Verification items for this drawing (mm, ordinates from the low corner). A direction names the side the tool comes from. Coordinates: 2 decimals unless noted, no trailing zeros. Write each loop counter-clockwise with the first axis right and the second up, starting at its lowest first coordinate (ties: lowest second). Pieces come first, ordered by that corner, then holes.
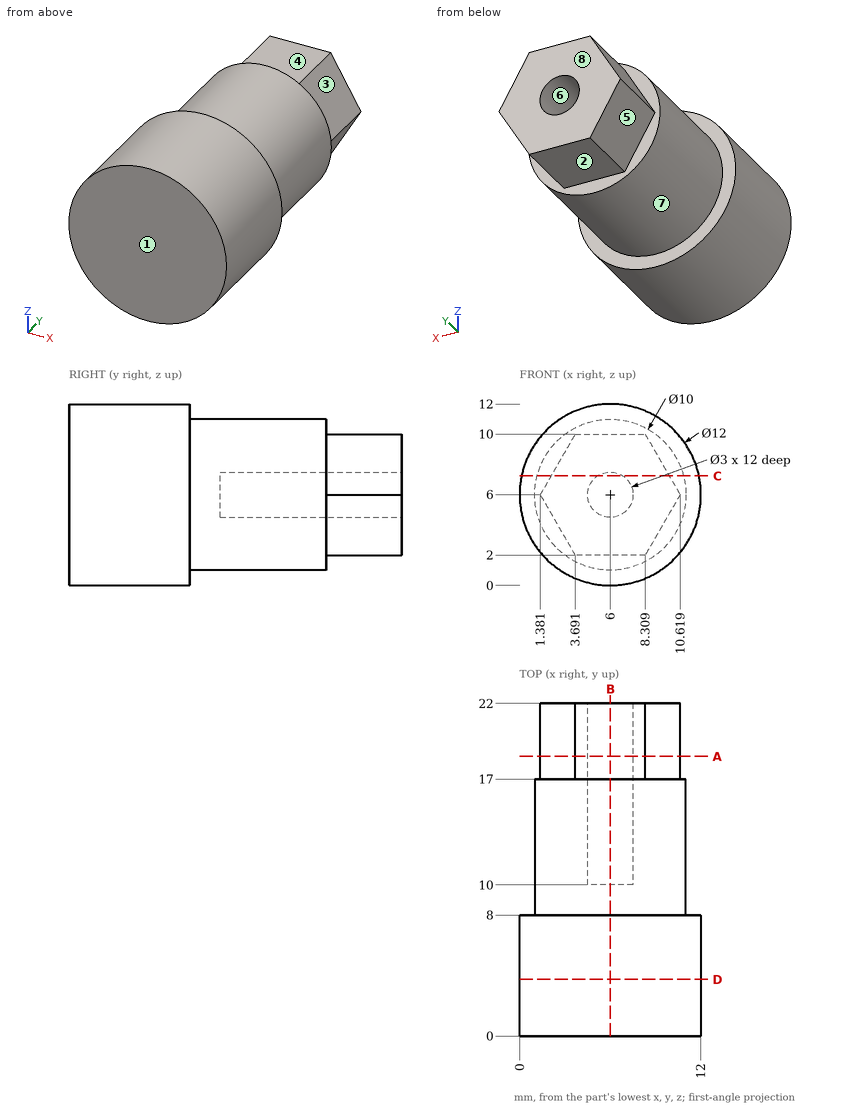
1. Sectioned sample at C-C, the plane z = 7.25. Record the boundary of the cut face in (x, y), and give its area (3 significant figures).
Computed values:
outline: (0.13, 0) - (11.87, 0) - (11.87, 8) - (10.84, 8) - (10.84, 17) - (9.9, 17) - (9.9, 22) - (6.83, 22) - (6.83, 10) - (5.17, 10) - (5.17, 22) - (2.1, 22) - (2.1, 17) - (1.16, 17) - (1.16, 8) - (0.13, 8) - close
area: 200 mm2
2. Thickness scan on line 1 along Z through (x, y) = (6, 16); line 2 along Z through (x, y) = (6, 17.75). Record the ranges inside material, lowest first.
Computed values:
line 1: z = 1 to 4.5, 7.5 to 11
line 2: z = 2 to 4.5, 7.5 to 10
3. Draft check along X on the marked faces 5, 6, 7 and 8. Enter one of: released by +X, released by -X, zero draft, split by the parting line, or undercut.
Computed values:
face 5: released by -X
face 6: undercut
face 7: split by the parting line
face 8: zero draft
4. Sectioned sample at B-B, the plane x = 6. Record the boundary of the cut face in (y, z), and give its area (3 significant figures).
Computed values:
outline: (0, 0) - (8, 0) - (8, 1) - (17, 1) - (17, 2) - (22, 2) - (22, 4.5) - (10, 4.5) - (10, 7.5) - (22, 7.5) - (22, 10) - (17, 10) - (17, 11) - (8, 11) - (8, 12) - (0, 12) - close
area: 190 mm2
5. Sectioned sample at A-A, the plane y = 18.5. Record the boundary of the cut face in (x, z).
Computed values:
outline: (1.38, 6) - (3.69, 2) - (8.31, 2) - (10.62, 6) - (8.31, 10) - (3.69, 10) - close; hole circle Ø3 at (6, 6)
6. Access from +Z, -Z, +X, -X, +Y, -Y to the whole of each face (thin tool, end or side, straight path). Record for the marked faces 1, 2, 3 and 4.
Computed values:
face 1: +Z, -Z, +X, -X, -Y
face 2: -Z, +X, -X, +Y
face 3: +Z, +X, +Y
face 4: +Z, +X, -X, +Y
7. Sectioned sample at D-D, the plane y = 3.75. Record the boundary of the cut face in (x, z), and give its area (3 significant figures).
Computed values:
outline: circle Ø12 at (6, 6)
area: 113 mm2
8. Gauge pin test, flat ends, axial feed: pin 1 Ø2.5 at (x, y) = (6.5, 18.5) entering from -Z; pin 2 Ø1.4 at (x, y) = (5, 20) entering from +Z; pin 3 Ø4 at (y, z) = (15, 2.5) entering from +X; pin 4 Ø4 at (x, z) = (6, 6) entering from -Y. Record the tip position at first contact, or that the pin passes through.
Computed values:
pin 1: stops at z = 2
pin 2: stops at z = 10
pin 3: stops at x = 10.77
pin 4: stops at y = 0
